Part model, mm, in its own coordinate system. Give positions to 0.01 mm unless a question says otherwise; leave off trailing zeros. Write each loop counter-clockwise with the first axis right and the second up, starting at its lowest first coordinate (ties: lowest second). Pieces come first, ordered by that corner, then holes. Notation, with made-up numbers: (11, 41.25) - (23, 41.25) arc R25 cw to (23, 68.25) - close; hole circle Ø10 at (31, 81.5). An arc over 180 degrees is marked (long way). Answer in a Markdown table with one row per item. Add a question column.
1. Band-saw the part on D-D on z = -36.5. Write the cut outline in (x, y).
2. Drop flat-ended pins along their axis: pin 1 Ø20 at (x, y) = (85, 40) entering from -Z; pin 2 Ø16 at (x, y) = (85, 0) entering from -Z. Give the stop position or say it passes through.
3. Probe line 1 along Y through (x, z) = (85, -29); line 2 along Y through (x, z) = (-20, -32); line 3 along X through (y, z) = (-32.5, -35). List the from-to ranges inside material, lowest first.
4. Band-saw the part on B-B on y = -40. Write the cut outline in (x, z), plus the area to 3 significant figures.
5. Band-saw the part on C-C on y = 0. Write the cut outline in (x, z), plus the area to 3 significant figures.
6. Band-saw the part on A-A on x = -20. Write the cut outline in (y, z), plus the area to 3 significant figures.
7. Pull direction X, two halves, no side cores. Call faces 1 (the cylindrical face through (-30.161, -4.213, -25.35)), 2 (the flat face through (-125, -1, -25)), 3 (the flat face through (-2, 1, -50)), 4 (the cylindrical face through (76.654, 2.628, -25.35)): released by +X, released by -X, zero draft, split by the parting line, or undercut.
```python
from build123d import *

# Parameters (mm, degrees)
SKETCH1_W                  = 250
SKETCH1_H                  = 120
BOSS_EXTRUDE1_DEPTH        = 50
F_22_0_22_DIAMETER_HOLE1_D = 22
M20_TAPPED_HOLE1_D         = 17.5
LPATTERN1_COUNT            = 2
LPATTERN1_PITCH            = 40
LPATTERN1_COL_COUNT        = 2
LPATTERN1_COL_PITCH        = 40


with BuildPart() as part:
    # Sketch1 → Boss-Extrude1 (new body)
    with BuildSketch(Plane.XY):
        Rectangle(SKETCH1_W, SKETCH1_H)
    extrude(amount=-BOSS_EXTRUDE1_DEPTH)

    # Ø22.0 (22) Diameter Hole1 (through all)
    with Locations(Plane.XY):
        with Locations((-20, 0)):
            Hole(F_22_0_22_DIAMETER_HOLE1_D / 2)

    # M20 Tapped Hole1 (through all)
    with Locations(Plane.XY):
        with Locations((85, 0)):
            m20_tapped_hole1 = Hole(M20_TAPPED_HOLE1_D / 2)

    # LPattern1: M20 Tapped Hole1 ×2
    with Locations(*[(0, -i * LPATTERN1_PITCH, 0) for i in range(1, LPATTERN1_COUNT)]):
        add(m20_tapped_hole1, mode=Mode.SUBTRACT)

    # LPattern1 col: M20 Tapped Hole1 ×2
    with Locations(*[(0, i * LPATTERN1_COL_PITCH, 0) for i in range(1, LPATTERN1_COL_COUNT)]):
        add(m20_tapped_hole1, mode=Mode.SUBTRACT)


solid = part.part
```
Values:
| question | item | result |
|---|---|---|
| 1 | outline | (-125, -60) - (125, -60) - (125, 60) - (-125, 60) - close; hole circle Ø22 at (-20, 0); hole circle Ø17.5 at (85, -40); hole circle Ø17.5 at (85, 0); hole circle Ø17.5 at (85, 40) |
| 2 | pin 1 | stops at z = -50 |
| 2 | pin 2 | passes through |
| 3 | line 1 | y = -60 to -48.75, -31.25 to -8.75, 8.75 to 31.25, 48.75 to 60 |
| 3 | line 2 | y = -60 to -11, 11 to 60 |
| 3 | line 3 | x = -125 to 80.49, 89.51 to 125 |
| 4 | outline | (-125, -50) - (76.25, -50) - (76.25, 0) - (-125, 0) - close; (93.75, -50) - (125, -50) - (125, 0) - (93.75, 0) - close |
| 4 | area | 11,600 mm² |
| 5 | outline | (-125, -50) - (-31, -50) - (-31, 0) - (-125, 0) - close; (-9, -50) - (76.25, -50) - (76.25, 0) - (-9, 0) - close; (93.75, -50) - (125, -50) - (125, 0) - (93.75, 0) - close |
| 5 | area | 10,500 mm² |
| 6 | outline | (-60, -50) - (-11, -50) - (-11, 0) - (-60, 0) - close; (11, -50) - (60, -50) - (60, 0) - (11, 0) - close |
| 6 | area | 4,900 mm² |
| 7 | face 1 | undercut |
| 7 | face 2 | released by -X |
| 7 | face 3 | zero draft |
| 7 | face 4 | undercut |
